Geometry: final body of the model. Coordinates: model frame, mm. Give positions to 0.01 mm unless a question says otherwise; leave off trailing zeros. Write each loop counter-clockwise with the first axis right and the second up, starting at its lowest first coordinate (ties: lowest second). Pieces come first, ordered by that corner, then holes.
```python
from build123d import *

# Parameters (mm, degrees)
F0_R     = 26
F1_DEPTH = 138


with BuildPart() as f1:
    # F0 (on Top) → F1 (new body)
    with BuildSketch(Plane.XY):
        Circle(F0_R)
        with BuildLine():
            ThreePointArc((16.704727, -17.232298), (16.478129, -17.449105), (16.248718, -17.662932))
            ThreePointArc((16.248718, -17.662932), (9.184402, -22.173109), (1, -23.979158))
            ThreePointArc((1, -23.979158), (0, -24), (-1, -23.979158))
            ThreePointArc((-1, -23.979158), (-9.184402, -22.173109), (-16.248718, -17.662932))
            ThreePointArc((-16.248718, -17.662932), (-16.970563, -16.970563), (-17.662932, -16.248718))
            ThreePointArc((-17.662932, -16.248718), (-22.173109, -9.184402), (-23.979158, -1))
            ThreePointArc((-23.979158, -1), (-24, 0), (-23.979158, 1))
            ThreePointArc((-23.979158, 1), (-22.173109, 9.184402), (-17.662932, 16.248718))
            ThreePointArc((-17.662932, 16.248718), (-16.970563, 16.970563), (-16.248718, 17.662932))
            ThreePointArc((-16.248718, 17.662932), (-9.184402, 22.173109), (-1, 23.979158))
            ThreePointArc((-1, 23.979158), (0, 24), (1, 23.979158))
            ThreePointArc((1, 23.979158), (9.184402, 22.173109), (16.248718, 17.662932))
            ThreePointArc((16.248718, 17.662932), (16.970563, 16.970563), (17.662932, 16.248718))
            ThreePointArc((17.662932, 16.248718), (22.173109, 9.184402), (23.979158, 1))
            ThreePointArc((23.979158, 1), (23.994789, 0.500109), (24, 0))
            ThreePointArc((24, 0), (23.994789, -0.500109), (23.979158, -1))
            ThreePointArc((23.979158, -1), (22.291296, -8.893714), (18.081746, -15.781332))
            ThreePointArc((18.081746, -15.781332), (17.40836, -16.521168), (16.704727, -17.232298))
        make_face(mode=Mode.SUBTRACT)
        with BuildLine():
            ThreePointArc((9.215691, -7.685769), (8.514268, -8.456195), (7.74866, -9.162874))
            Line((7.74866, -9.162874), (16.248718, -17.662932))
            ThreePointArc((16.248718, -17.662932), (16.478129, -17.449105), (16.704727, -17.232298))
            ThreePointArc((16.704727, -17.232298), (17.40836, -16.521168), (18.081746, -15.781332))
            Line((18.081746, -15.781332), (9.215691, -7.685769))
        make_face()
        with BuildLine():
            Line((-16.248718, -17.662932), (-7.74866, -9.162874))
            ThreePointArc((-7.74866, -9.162874), (-8.485281, -8.485281), (-9.162874, -7.74866))
            Line((-9.162874, -7.74866), (-17.662932, -16.248718))
            ThreePointArc((-17.662932, -16.248718), (-16.970563, -16.970563), (-16.248718, -17.662932))
        make_face()
        with BuildLine():
            ThreePointArc((1, -11.958261), (4.592201, -11.086554), (7.74866, -9.162874))
            ThreePointArc((7.74866, -9.162874), (8.514268, -8.456195), (9.215691, -7.685769))
            ThreePointArc((9.215691, -7.685769), (11.102204, -4.554236), (11.958261, -1))
            ThreePointArc((11.958261, -1), (11.989561, -0.500435), (12, 0))
            ThreePointArc((12, 0), (11.989561, 0.500435), (11.958261, 1))
            ThreePointArc((11.958261, 1), (11.086554, 4.592201), (9.162874, 7.74866))
            ThreePointArc((9.162874, 7.74866), (8.485281, 8.485281), (7.74866, 9.162874))
            ThreePointArc((7.74866, 9.162874), (4.592201, 11.086554), (1, 11.958261))
            ThreePointArc((1, 11.958261), (0, 12), (-1, 11.958261))
            ThreePointArc((-1, 11.958261), (-4.592201, 11.086554), (-7.74866, 9.162874))
            ThreePointArc((-7.74866, 9.162874), (-8.485281, 8.485281), (-9.162874, 7.74866))
            ThreePointArc((-9.162874, 7.74866), (-11.086554, 4.592201), (-11.958261, 1))
            ThreePointArc((-11.958261, 1), (-12, 0), (-11.958261, -1))
            ThreePointArc((-11.958261, -1), (-11.086554, -4.592201), (-9.162874, -7.74866))
            ThreePointArc((-9.162874, -7.74866), (-8.485281, -8.485281), (-7.74866, -9.162874))
            ThreePointArc((-7.74866, -9.162874), (-4.592201, -11.086554), (-1, -11.958261))
            ThreePointArc((-1, -11.958261), (0, -12), (1, -11.958261))
        make_face()
        with BuildLine():
            ThreePointArc((-7.177134, -7.177134), (-10.15, 0), (-7.177134, 7.177134))
            ThreePointArc((-7.177134, 7.177134), (-5.22891, 8.699483), (-2.970415, 9.705624))
            ThreePointArc((-2.970415, 9.705624), (-1.501735, 10.038291), (0, 10.15))
            ThreePointArc((0, 10.15), (9.377377, -3.884237), (-7.177134, -7.177134))
        make_face(mode=Mode.SUBTRACT)
        with BuildLine():
            Line((1, -23.979158), (1, -11.958261))
            ThreePointArc((1, -11.958261), (0, -12), (-1, -11.958261))
            Line((-1, -11.958261), (-1, -23.979158))
            ThreePointArc((-1, -23.979158), (0, -24), (1, -23.979158))
        make_face()
        with BuildLine():
            ThreePointArc((12, 0), (11.989561, -0.500435), (11.958261, -1))
            Line((11.958261, -1), (23.979158, -1))
            ThreePointArc((23.979158, -1), (23.994789, -0.500109), (24, 0))
            ThreePointArc((24, 0), (23.994789, 0.500109), (23.979158, 1))
            Line((23.979158, 1), (11.958261, 1))
            ThreePointArc((11.958261, 1), (11.989561, 0.500435), (12, 0))
        make_face()
        with BuildLine():
            ThreePointArc((7.74866, 9.162874), (8.485281, 8.485281), (9.162874, 7.74866))
            Line((9.162874, 7.74866), (17.662932, 16.248718))
            ThreePointArc((17.662932, 16.248718), (16.970563, 16.970563), (16.248718, 17.662932))
            Line((16.248718, 17.662932), (7.74866, 9.162874))
        make_face()
        with BuildLine():
            ThreePointArc((-1, 11.958261), (0, 12), (1, 11.958261))
            Line((1, 11.958261), (1, 23.979158))
            ThreePointArc((1, 23.979158), (0, 24), (-1, 23.979158))
            Line((-1, 23.979158), (-1, 11.958261))
        make_face()
        with BuildLine():
            Line((-17.662932, 16.248718), (-9.162874, 7.74866))
            ThreePointArc((-9.162874, 7.74866), (-8.485281, 8.485281), (-7.74866, 9.162874))
            Line((-7.74866, 9.162874), (-16.248718, 17.662932))
            ThreePointArc((-16.248718, 17.662932), (-16.970563, 16.970563), (-17.662932, 16.248718))
        make_face()
        with BuildLine():
            Line((-23.979158, -1), (-11.958261, -1))
            ThreePointArc((-11.958261, -1), (-12, 0), (-11.958261, 1))
            Line((-11.958261, 1), (-23.979158, 1))
            ThreePointArc((-23.979158, 1), (-24, 0), (-23.979158, -1))
        make_face()
    extrude(amount=F1_DEPTH)


solid = f1.part
```
Item 1: Section C-C, the plane z = 31. State how many separate pieces and enclosed holes the cut face has, plus the area to 3 significant figures.
Found:
separate pieces: 1
enclosed holes: 9
area: 639 mm2
Item 2: Section A-A, the plane y = -20.5. Return the cut outline in (x, z).
Found:
outline: (-15.99, 0) - (-12.48, 0) - (-12.48, 138) - (-15.99, 138) - close; (-1, 0) - (1, 0) - (1, 138) - (-1, 138) - close; (12.48, 0) - (15.99, 0) - (15.99, 138) - (12.48, 138) - close
Item 3: Section D-D, the plane y = 21.5. Return the cut outline in (x, z).
Found:
outline: (-14.62, 0) - (-10.67, 0) - (-10.67, 138) - (-14.62, 138) - close; (-1, 0) - (1, 0) - (1, 138) - (-1, 138) - close; (10.67, 0) - (14.62, 0) - (14.62, 138) - (10.67, 138) - close
Item 4: Pin query (flat end, axial travel): pin 1 Ø13 at (x, z) = (21, 52.5) entering from -Y; pin 2 Ø13 at (y, z) = (-16, 61.5) entering from +X; pin 3 Ø2 at (y, z) = (9, 106.5) entering from +X; pin 4 Ø6 at (x, y) = (1.5, 8.5) entering from -Z. Return the tip coordinate at first contact, or that it passes through.
Found:
pin 1: stops at y = -21.58
pin 2: stops at x = 24.2
pin 3: stops at x = 24.74
pin 4: stops at z = 0
Item 5: Line query: L1, parallel to Y at x = 0, z = 105.5; L2, parallel to X at y = 10.5, z = 78; L3, parallel to Y at x = -13, z = 103. Output: solid intervals per line, ascending.
Found:
L1: y = -26 to -10.15, 10.15 to 26
L2: x = -23.79 to -21.58, -11.91 to -9.09, -5.81 to 5.81, 9.09 to 11.91, 21.58 to 23.79
L3: y = -22.52 to -20.17, -14.41 to -11.59, -1 to 1, 11.59 to 14.41, 20.17 to 22.52
Item 6: Section B-B, the plane y = 14.5. Return the cut outline in (x, z), plus the area to 3 significant figures.
Found:
outline: (-21.58, 0) - (-19.12, 0) - (-19.12, 138) - (-21.58, 138) - close; (-15.91, 0) - (-13.09, 0) - (-13.09, 138) - (-15.91, 138) - close; (-1, 0) - (1, 0) - (1, 138) - (-1, 138) - close; (13.09, 0) - (15.91, 0) - (15.91, 138) - (13.09, 138) - close; (19.12, 0) - (21.58, 0) - (21.58, 138) - (19.12, 138) - close
area: 1,730 mm2
